Design review of the part built by this model. Coordinates are the model's own, in mm. Round coordinates to 2 decimals unless told otherwise and drop trailing zeros. Order: outer loops, then holes, each group sorted by start corner. A loop starts at its lowest first (then second) coordinate and runs counter-clockwise, first axis right, second up. Notation, with made-up numbers: M 24,62.5 L 43,62.5 A24 ccw 43,91.5 Z; hole C 19.25,76 d1. An arc over 180 degrees is marked long. Write each question's results on one line, items separated by ' | '. Start each with the question number.
Item 1: Clearance check with a flat-ended pin moving along its axis: pin 1 (25 mm diameter, centred on y = 90.5, z = 27.5, fed in from -X). State where the tip first meets the part, or that it passes through.
Item 2: Take a section at D-D, the plane z = 27.5. Write out the cut boundary in (x, y).
Item 3: Take a section at B-B, the plane y = 15. Write out the cut boundary in (x, z), plus the area to 3 significant figures.
Item 4: Take a section at C-C, the plane x = -3.5. Write out the cut boundary in (y, z), plus the area to 3 significant figures.
Item 5: Wall thickness on line 1 (Z direction, x = -4.5, y = 90); line 2 (Y direction, x = 2.5, z = 73); line 3 (Y direction, x = 8, z = 12.5): over which ranges is each line inside the solid? List them lowest first. Write a range as [from, to].
Item 6: Take a section at A-A, the plane z = 73. Write out the cut boundary in (x, y), plus the area to 3 significant figures.
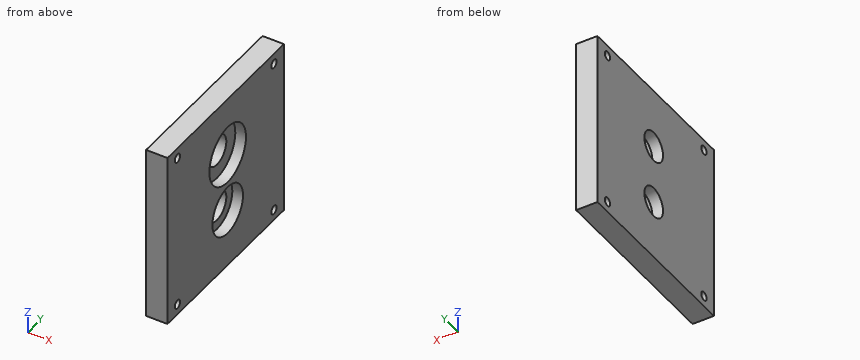
```python
from build123d import *

# Parameters (mm, degrees)
SKETCH1_W           = 20
SKETCH1_H           = 166
BOSS_EXTRUDE1_DEPTH = 175
SKETCH2_R           = 14
CUT_EXTRUDE1_DEPTH  = 175
SKETCH3_R           = 27.5
SKETCH3_R_2         = 23
CUT_EXTRUDE2_DEPTH  = 10
SKETCH4_R           = 4
CUT_EXTRUDE3_DEPTH  = 21


with BuildPart() as part:
    # Sketch1 → Boss-Extrude1 (new body)
    with BuildSketch(Plane(origin=(0, 0, 0), x_dir=(1, 0, 0), z_dir=(0, 1, 0))):
        Rectangle(SKETCH1_W, SKETCH1_H)
    extrude(amount=BOSS_EXTRUDE1_DEPTH)

    # Sketch2 → Cut-Extrude1 (cut)
    with BuildSketch(Plane(origin=(10, 0, 0), x_dir=(0, 0, -1), z_dir=(1, 0, 0))):
        with Locations((-27.5, 90.5)):
            Circle(SKETCH2_R)
        with Locations((28, 90.5)):
            Circle(SKETCH2_R)
    extrude(amount=-CUT_EXTRUDE1_DEPTH, mode=Mode.SUBTRACT)

    # Sketch3 → Cut-Extrude2 (cut)
    with BuildSketch(Plane(origin=(10, 0, 0), x_dir=(0, 0, -1), z_dir=(1, 0, 0))):
        with Locations((-27.5, 90.5)):
            Circle(SKETCH3_R)
        with Locations((28, 90.5)):
            Circle(SKETCH3_R_2)
    extrude(amount=-CUT_EXTRUDE2_DEPTH, mode=Mode.SUBTRACT)

    # Sketch4 → Cut-Extrude3 (cut, through all)
    with BuildSketch(Plane(origin=(10, 0, 0), x_dir=(0, 0, -1), z_dir=(1, 0, 0))):
        with Locations((73, 160)):
            Circle(SKETCH4_R)
        with Locations((73, 15)):
            Circle(SKETCH4_R)
        with Locations((-73, 15)):
            Circle(SKETCH4_R)
        with Locations((-73, 160)):
            Circle(SKETCH4_R)
    extrude(amount=-CUT_EXTRUDE3_DEPTH, mode=Mode.SUBTRACT)


solid = part.part
```
Results list:
1) pin 1: through
2) outline: M -10,0 L 10,0 L 10,63 L 0,63 L 0,76.5 L -10,76.5 Z; M -10,104.5 L 0,104.5 L 0,118 L 10,118 L 10,175 L -10,175 Z
3) outline: M -10,-83 L 10,-83 L 10,-77 L -10,-77 Z; M -10,-69 L 10,-69 L 10,69 L -10,69 Z; M -10,77 L 10,77 L 10,83 L -10,83 Z | area: 3,000 mm²
4) outline: M 0,-83 L 175,-83 L 175,83 L 0,83 Z; hole C 15,-73 d8; hole C 15,73 d8; hole C 90.5,-28 d28; hole C 90.5,27.5 d28; hole C 160,-73 d8; hole C 160,73 d8 | area: 27,600 mm²
5) line 1: [-83, -41.99], [-14.01, 13.51], [41.49, 83] | line 2: [0, 11], [19, 156], [164, 175] | line 3: [0, 67.45], [113.55, 175]
6) outline: M -10,0 L 10,0 L 10,11 L -10,11 Z; M -10,19 L 10,19 L 10,156 L -10,156 Z; M -10,164 L 10,164 L 10,175 L -10,175 Z | area: 3,180 mm²
